Part model, mm, in its own coordinate system. Face numbers are marked on the shaded views. A direction names the side the tool comes from. Coordinates: 2 decimals unless noted, no trailing zeros. Loops run counter-clockwise (first coordinate to the right, second up) from the corner with the lowest first, then second, coordinate; pieces in that order, holes last. Notation, with made-up numbers: (4.25, -33.5) - (43.25, -33.5) arc R11 ccw to (43.25, -21.5) - close; hole circle Ø2 at (11, 51). An arc over 180 degrees is marked (long way). Use a Markdown table: item, result. Add a question column.
1. Band-saw the part on C-C, the plane y = 30. Give the cut face in (x, z).
2. Drop flat-ended pins along their axis: pin 1 (1 mm diameter, centred on x = 76.5, z = -46, fed in from +Y); pin 2 (2 mm diameter, centred on x = 2.5, z = -2.5, fed in from +Y). Give the stop position or say it passes through.
3. 3-axis set-ups, long thin cutter, end or side, ignore diameter. For the marked faces 5 and 6: which of +Z, -Z, +X, -X, +Y, -Y reach the whole face in a straight line?
4. Pull direction X, two halves, no side cores. Call the marked faces 1, 2, 3 and 4: pulls with the +X half, pulls with the -X half, needs draft (parallel to the pull), parting line crosses it, or undercut.
5. Band-saw the part on B-B, the plane y = 43. Give the cut face in (x, z).
6. Wall check: probe 1 along Z at (x, y) = (162, 49); probe 2 along X at (y, z) = (51.65, -3); probe 3 along X at (y, z) = (51.5, -42.5). Give the ranges that are in metal, low to high. Write a range as [from, to].
7. Band-saw the part on D-D, the plane z = -3. Give the cut face in (x, y).
8. Band-saw the part on A-A, the plane z = -34.5. Give the cut face in (x, y).
Autodesk Inventor part; units mm, degrees
ref_plane "YZ Plane" through (0, 0, 0) normal (1, 0, 0) x (0, 1, 0)
ref_plane "XZ Plane" through (0, 0, 0) normal (0, 1, 0) x (-1, 0, 0)
ref_plane "XY Plane" through (0, 0, 0) normal (0, 0, 1) x (1, 0, 0)
sketch "草圖2" plane through (0, 0, 0) normal (0, 1, 0) x (-1, 0, 0)
  line L0 (0, 0) -> (-165, 0)
  line L1 (-165, 0) -> (-165, -95)
  line L2 (-165, -95) -> (0, -95)
  line L3 (0, -95) -> (0, 0)
  dimension "d1" = 95
  dimension "d2" = 165
extrude "擠出1" add sketch "草圖2" along normal blind 3
sketch "草圖3" plane through (0, 3, 0) normal (0, 1, 0) x (1, 0, 0)
  line L0 (5, 90) -> (160, 90)
  line L1 (160, 90) -> (160, 5)
  line L2 (160, 5) -> (5, 5)
  line L3 (5, 5) -> (5, 90)
  line L4 (165, 95) -> (0, 95)
  line L5 (165, 0) -> (165, 95)
  line L6 (0, 0) -> (165, 0)
  line L7 (0, 95) -> (0, 0)
  dimension "d5" = 5
  dimension "d6" = 5
  dimension "d7" = 5
  dimension "d8" = 5
extrude "擠出2" add sketch "草圖3" along normal blind 50
sketch "草圖4" plane through (0, 53, 0) normal (0, 1, 0) x (1, 0, 0)
  circle A0 centre (3, 92) radius 2
  line L0 (165, 95) -> (0, 95)
  line L1 (0, 95) -> (0, 0)
  circle A1 centre (3, 3) radius 2
  line L2 (0, 0) -> (165, 0)
  circle A2 centre (162, 3) radius 2
  line L3 (165, 0) -> (165, 95)
  circle A3 centre (162, 92) radius 2
  dimension "d11" = 4
  dimension "d12" = 3
  dimension "d13" = 3
  dimension "d14" = 4
  dimension "d15" = 3
  dimension "d16" = 3
  dimension "d17" = 4
  dimension "d18" = 3
  dimension "d19" = 3
  dimension "d20" = 4
  dimension "d21" = 3
  dimension "d22" = 3
extrude "擠出3" cut sketch "草圖4" against normal blind 5 contours A0 | A1 | A2 | A3
sketch "草圖7" plane through (5, 3, -5) normal (1, 0, 0) x (0, 0, -1)
  line L0 (85, 50) -> (0, 50)
  line L1 (0, 50) -> (0, 0)
  line L2 (0, 0) -> (85, 0)
  line L3 (85, 0) -> (85, 50)
  line L4 (0, 50) -> (85, 50)
  line L5 (85, 0) -> (85, 50)
  line L6 (85, 0) -> (0, 0)
  line L7 (0, 0) -> (0, 50)
  point P0 (-5, -3)
extrude "擠出4" add sketch "草圖7" along normal blind 3
sketch "草圖8" plane through (0, 0, -95) normal (-1, 0, 0) x (0, 0, 1)
  circle A0 centre (34.5, 30) radius 8.5
  circle A1 centre (60.5, 30) radius 8.5
  line L0 (0, 0) -> (95, 0)
  line L1 (0, 0) -> (0, 53)
  dimension "d27" = 17
  dimension "d28" = 17
  dimension "d29" = 26
  dimension "d30" = 30
  dimension "d31" = 30
  dimension "d32" = 34.5
extrude "擠出5" cut sketch "草圖8" against normal blind 60
sketch "草圖9" plane through (0, 0, 0) normal (0, 0, 1) x (1, 0, 0)
  line L0 (95, 26) -> (155, 26)
  line L1 (155, 26) -> (155, 6)
  line L2 (155, 6) -> (95, 6)
  line L3 (95, 6) -> (95, 26)
  line L4 (160, 3) -> (8, 3)
  line L5 (165, 0) -> (165, 53)
  point P0 (0, 0)
  dimension "d35" = 3
  dimension "d38" = 20
  dimension "d39" = 60
  dimension "d40" = 10
extrude "擠出6" cut sketch "草圖9" against normal blind 10
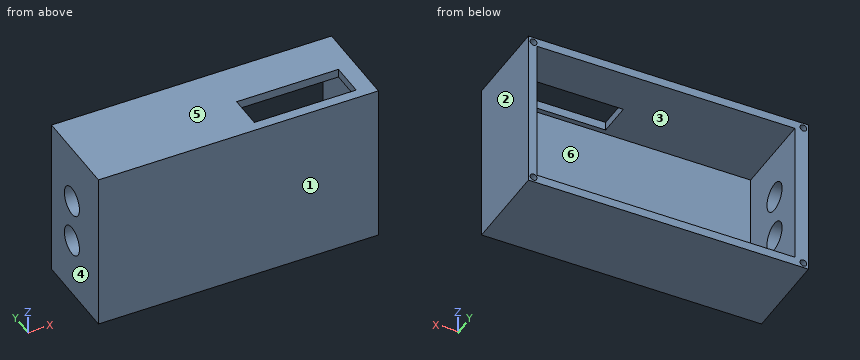
Geometry check:
| question | item | result |
|---|---|---|
| 1 | outline | (0, -95) - (165, -95) - (165, 0) - (0, 0) - (0, -26) - (8, -26) - (8, -5) - (160, -5) - (160, -90) - (8, -90) - (8, -69) - (0, -69) - close; (0, -52) - (8, -52) - (8, -43) - (0, -43) - close |
| 2 | pin 1 | stops at y = 3 |
| 2 | pin 2 | stops at y = 48 |
| 3 | face 5 | +Z, +X, -X, +Y, -Y |
| 3 | face 6 | +Y |
| 4 | face 1 | needs draft |
| 4 | face 2 | pulls with the +X half |
| 4 | face 3 | undercut |
| 4 | face 4 | pulls with the -X half |
| 5 | outline | (0, -95) - (165, -95) - (165, 0) - (0, 0) - close; hole (8, -90) - (160, -90) - (160, -5) - (8, -5) - close |
| 6 | probe 1 | z = [-95, -94], [-90, -5], [-1, 0] |
| 6 | probe 2 | x = [0, 1], [5, 160], [164, 165] |
| 6 | probe 3 | x = [0, 8], [160, 165] |
| 7 | outline | (0, 0) - (165, 0) - (165, 53) - (164, 53) - (164, 48) - (160, 48) - (160, 53) - (5, 53) - (5, 48) - (1, 48) - (1, 53) - (0, 53) - close; hole (95, 6) - (155, 6) - (155, 26) - (95, 26) - close |
| 8 | outline | (0, 0) - (165, 0) - (165, 53) - (160, 53) - (160, 3) - (8, 3) - (8, 21.5) - (0, 21.5) - close; (0, 38.5) - (8, 38.5) - (8, 53) - (0, 53) - close |
